```python
from build123d import *

# Parameters (mm, degrees)
F1_DEPTH = 63.5
F2_DEPTH = 25.4
F0_W     = 24.304205
F0_H     = 19.05
F3_DEPTH = 25.4
F5_DEPTH = 7.9375
F6_R     = 6.35


with BuildPart() as f1:
    # F0 (on Front) → F1 (new body, symmetric)
    with BuildSketch(Plane.XZ):
        Polygon((-41.275, 9.525), (-41.275, -9.525), (41.275, -9.525), (41.275, 9.525), (22.225, 9.525), align=None)
    extrude(amount=F1_DEPTH, both=True)

    # F0 (on Front) → F2 (join, symmetric)
    with BuildSketch(Plane.XZ):
        with BuildLine():
            Line((22.225, 9.525), (41.275, 9.525))
            Line((41.275, 9.525), (41.275, 27.0002))
            ThreePointArc((41.275, 27.0002), (45.92468, 38.22552), (57.15, 42.8752))
            Line((57.15, 42.8752), (61.420795, 42.8752))
            Line((61.420795, 42.8752), (61.420795, 61.9252))
            Line((61.420795, 61.9252), (57.15, 61.9252))
            ThreePointArc((57.15, 61.9252), (32.454296, 51.695904), (22.225, 27.0002))
            Line((22.225, 27.0002), (22.225, 9.525))
        make_face()
    extrude(amount=F2_DEPTH, both=True)

    # F0 (on Front) → F3 (join, symmetric)
    with BuildSketch(Plane.XZ):
        with Locations((73.572897, 52.4002)):
            Rectangle(F0_W, F0_H)
    extrude(amount=F3_DEPTH, both=True)

    # F0 (on Front) → F4 (revolve)
    with BuildSketch(Plane.XZ):
        Polygon((85.725, 66.675), (85.725, 61.9252), (85.725, 42.8752), (85.725, 38.1), (112.220795, 38.1), (112.220795, 66.675), align=None)
    revolve(axis=Axis((85.725, 0, 54.7751), (0, 0, -1)))

    # F0 (on Front) → F5 (join, symmetric)
    with BuildSketch(Plane.XZ):
        with BuildLine():
            add(Edge.make_bspline(
                [(-41.275, 9.525), (-26.246125, 52.973336), (22.107758, 63.136719), (61.420795, 61.9252)],
                knots=[0, 0, 0, 0, 115.291835, 115.291835, 115.291835, 115.291835], degree=3))
            Line((-41.275, 9.525), (22.225, 9.525))
            Line((22.225, 9.525), (22.225, 27.0002))
            ThreePointArc((22.225, 27.0002), (32.454296, 51.695904), (57.15, 61.9252))
            Line((57.15, 61.9252), (61.420795, 61.9252))
        make_face()
    extrude(amount=F5_DEPTH, both=True)

    # F6
    f6_edges = [f1.edges().sort_by_distance(p)[0] for p in [
        (41.275, 63.5, 0),
        (-41.275, 63.5, 0),
        (-41.275, -63.5, 0),
        (41.275, -63.5, 0),
    ]]
    fillet(f6_edges, radius=F6_R)


solid = f1.part
```
For this review, take the finished solid that the model builds, in its own axes (mm). A direction names the side the tool comes from. Coordinates: 2 decimals unless noted, no trailing zeros. Write each loop counter-clockwise with the first axis right and the second up, starting at its lowest first coordinate (ties: lowest second). Pieces come first, ordered by that corner, then holes. Notation, with made-up numbers: (22, -1) - (67, -1) arc R9 cw to (67, 13) - close; hole circle Ø5 at (61.25, -14.5). An arc over 180 degrees is marked (long way). Answer in a Markdown table with one row per item. Add a question column.
Q1. We need section C-C, the plane x = 63. State the section outline as (y, z) points (3 decimals), and give its area (3 significant figures).
Q2. We need section A-A, the plane z = -4. State the section outline as (x, y) points (3 decimals), and give its area (3 significant figures).
Q3. Tool access review of faces 1 (the flat face through (1, 35, 9.525)), 2 (the flat face through (59, 2, 42.875)), 3 (the flat face through (41.275, -1, 4)), 4 (the flat face through (22.225, -17, 18)): name each direction out of +Z, -Z, +X, -X, +Y, -Y from which nothing blocks a thin tool from reaching the whole face with its end or side.
Q4. For probe 1 along X at (y, z) = (-35.5, 2.5) (3 decimals); probe 2 along Z at (x, y) = (-24.5, 11.5) (3 decimals); probe 3 along Y at (x, z) = (55.5, 45), list the stretches that pass through material, from the lowest coordinate up.
Q5. We need section B-B, the plane y = -13.5. State the section outline as (x, z) points (3 decimals).
Q6. For P1, Ø10.5, axis at x = 65, y = -12.5, coming from the -Z side; P2, Ø5, axis at y = -16.5, z = 17.5, coming from the -X side (3 decimals); P3, Ø4, axis at y = 50.5, z = -1.5, coming from the +X side (3 decimals), all flat-tipped, find the tip position at first contact; note any pin that passes through.
Q7. We need section D-D, the plane x = 83. State the section outline as (y, z) points (3 decimals), and give its area (3 significant figures).
Answer list:
| question | item | result |
|---|---|---|
| 1 | outline | (-25.4, 42.875) - (-13.624, 42.875) - (-13.624, 38.1) - (13.624, 38.1) - (13.624, 42.875) - (25.4, 42.875) - (25.4, 61.925) - (13.624, 61.925) - (13.624, 66.675) - (-13.624, 66.675) - (-13.624, 61.925) - (-25.4, 61.925) - close |
| 1 | area | 1,230 mm2 |
| 2 | outline | (-41.275, -57.15) arc R6.35 ccw to (-34.925, -63.5) - (34.925, -63.5) arc R6.35 ccw to (41.275, -57.15) - (41.275, 57.15) arc R6.35 ccw to (34.925, 63.5) - (-34.925, 63.5) arc R6.35 ccw to (-41.275, 57.15) - close |
| 2 | area | 10,400 mm2 |
| 3 | face 1 | +Z, -X, +Y |
| 3 | face 2 | -Z |
| 3 | face 3 | -Z, +X, +Y, -Y |
| 3 | face 4 | +Z, -X, -Y |
| 4 | probe 1 | x = -41.275 to 41.275 |
| 4 | probe 2 | z = -9.525 to 9.525 |
| 4 | probe 3 | y = -25.4 to 25.4 |
| 5 | outline | (-41.275, -9.525) - (41.275, -9.525) - (41.275, 27) arc R15.875 cw to (57.15, 42.875) - (62.926, 42.875) - (62.926, 38.1) - (108.524, 38.1) - (108.524, 66.675) - (62.926, 66.675) - (62.926, 61.925) - (57.15, 61.925) arc R34.925 ccw to (22.225, 27) - (22.225, 9.525) - (-41.275, 9.525) - close |
| 6 | P1 | stops at z = 38.1 |
| 6 | P2 | stops at x = 22.225 |
| 6 | P3 | stops at x = 41.275 |
| 7 | outline | (-26.355, 38.1) - (26.355, 38.1) - (26.355, 66.675) - (-26.355, 66.675) - close |
| 7 | area | 1,510 mm2 |
